from build123d import *

# Parameters (mm, degrees)
SKETCH1_W                      = 132.1
SKETCH1_H                      = 36
BOSS_EXTRUDE1_DEPTH            = 44
CUT_EXTRUDE1_REACH             = 89.147
CUT_EXTRUDE2_REACH             = 89.147
SKETCH3_4_W                    = 23.05
SKETCH3_4_H                    = 12
SKETCH3_4_W_2                  = 52.5
SKETCH3_4_H_2                  = 26
CUT_EXTRUDE3_DEPTH             = 12.5
CUT_EXTRUDE6_DEPTH             = 7.5
CUT_EXTRUDE7_REACH             = 101.054
CUT_EXTRUDE8_REACH             = 137.7
SKETCH11_R                     = 2.55
CUT_EXTRUDE8_DIRECTION_2_REACH = 137.7
SKETCH11_6_R                   = 4.6
SKETCH11_6_R_2                 = 2.55
CUT_EXTRUDE10_DEPTH            = 2.2
CUT_EXTRUDE11_START            = 123.73
SKETCH11_7_R                   = 4.6
SKETCH11_7_R_2                 = 2.55
CUT_EXTRUDE11_DEPTH            = 2.2


with BuildPart() as part:
    # Sketch1 → Boss-Extrude1 (new body)
    with BuildSketch(Plane(origin=(0, 0, 0), x_dir=(1, 0, 0), z_dir=(0, 1, 0))):
        Rectangle(SKETCH1_W, SKETCH1_H)
        Polygon((-57.05, 14.5), (-57.05, -5.5), (20.85, -5.5), (20.85, -3.2), (26.85, 0.267693758), (32.85, -3.2), (33.05, -3.2), (33.05, 9.51), (32.85, 9.51), (26.85, 6.042306242), (20.85, 9.51), (20.85, 13), (-37.95, 13), (-37.95, 14.5), align=None, mode=Mode.SUBTRACT)
    extrude(amount=-BOSS_EXTRUDE1_DEPTH)

    # Cut-Extrude1: up to this face of the body (flat: up to its plane)
    cut_extrude1_end = Plane(part.part.faces().sort_by_distance((0, -22, 18))[0])
    # Sketch3 → Cut-Extrude1 (cut, up to the picked face)
    with BuildSketch(Plane(origin=(0, 0, -18), x_dir=(-1, 0, 0), z_dir=(0, 0, -1)), mode=Mode.PRIVATE) as cut_extrude1_sk1:
        Polygon((-60.48, -18), (-60.48, -44), (-20.85, -44), (-20.85, -29), (-38.35, -29), (-38.35, -22), (-46.35, -14), (-56.48, -14), align=None)
    cut_extrude1_tool1 = split(extrude(cut_extrude1_sk1.sketch, amount=-CUT_EXTRUDE1_REACH, mode=Mode.PRIVATE), bisect_by=cut_extrude1_end, keep=Keep.BOTH, mode=Mode.PRIVATE)
    add(cut_extrude1_tool1.solids().sort_by(Axis((43.76231, -31.789655, -18), (0, 0, 1)))[0], mode=Mode.SUBTRACT)

    # Cut-Extrude2: up to this face of the body (flat: up to its plane)
    cut_extrude2_end = Plane(part.part.faces().sort_by_distance((-18.1, -22, 5.5))[0])
    # Sketch3<4> → Cut-Extrude2 (cut, up to the picked face)
    with BuildSketch(Plane(origin=(0, 0, -18), x_dir=(-1, 0, 0), z_dir=(0, 0, -1)), mode=Mode.PRIVATE) as cut_extrude2_sk1:
        with Locations((20.075, -10.36)):
            Rectangle(SKETCH3_4_W, SKETCH3_4_H)
    cut_extrude2_tool1 = split(extrude(cut_extrude2_sk1.sketch, amount=-CUT_EXTRUDE2_REACH, mode=Mode.PRIVATE), bisect_by=cut_extrude2_end, keep=Keep.BOTH, mode=Mode.PRIVATE)
    # Sketch3<4> → Cut-Extrude2 (cut, up to the picked face)
    with BuildSketch(Plane(origin=(0, 0, -18), x_dir=(-1, 0, 0), z_dir=(0, 0, -1)), mode=Mode.PRIVATE) as cut_extrude2_sk2:
        with Locations((34.8, -31)):
            Rectangle(SKETCH3_4_W_2, SKETCH3_4_H_2)
    cut_extrude2_tool2 = split(extrude(cut_extrude2_sk2.sketch, amount=-CUT_EXTRUDE2_REACH, mode=Mode.PRIVATE), bisect_by=cut_extrude2_end, keep=Keep.BOTH, mode=Mode.PRIVATE)
    add(cut_extrude2_tool1.solids().sort_by(Axis((-20.075, -10.36, -18), (0, 0, 1)))[0], mode=Mode.SUBTRACT)
    add(cut_extrude2_tool2.solids().sort_by(Axis((-34.8, -31, -18), (0, 0, 1)))[0], mode=Mode.SUBTRACT)

    # Sketch4 → Cut-Extrude3 (cut)
    with BuildSketch(Plane.XY.offset(18)):
        Polygon((-61.05, -44), (-61.05, -18), (-57.05, -18), (-57.05, -14), (-35.05, -14), (-27.05, -22), (-27.05, -29), (-14.05, -29), (-5.05, -21.5), (20.85, -21.5), (20.85, -29), (20.85, -44), align=None)
    extrude(amount=-CUT_EXTRUDE3_DEPTH, mode=Mode.SUBTRACT)

    # Sketch7 → Cut-Extrude6 (cut)
    with BuildSketch(Plane.XZ.offset(29)):
        Polygon((20.85, 3.2), (23.35, 5.7), (23.35, 8), (29.35, 8), (28.95, 18), (20.85, 18), align=None)
    extrude(amount=-CUT_EXTRUDE6_DEPTH, mode=Mode.SUBTRACT)

    # Cut-Extrude7: up to this face of the body (flat: up to its plane)
    cut_extrude7_end = Plane(part.part.faces().sort_by_distance((33.05, -14.5, -3.155))[0])
    # Sketch10 → Cut-Extrude7 (cut, up to the picked face)
    with BuildSketch(Plane.ZY.offset(-20.85), mode=Mode.PRIVATE) as cut_extrude7_sk1:
        Polygon((-8.552306242, 0), (-6.042306242, 0), (-6.042306242, -2.51), align=None)
    cut_extrude7_tool1 = split(extrude(cut_extrude7_sk1.sketch, amount=-CUT_EXTRUDE7_REACH, mode=Mode.PRIVATE), bisect_by=cut_extrude7_end, keep=Keep.BOTH, mode=Mode.PRIVATE)
    # Sketch10 → Cut-Extrude7 (cut, up to the picked face)
    with BuildSketch(Plane.ZY.offset(-20.85), mode=Mode.PRIVATE) as cut_extrude7_sk2:
        Polygon((-0.267693758, 0), (-0.267693758, -2.51), (2.242306242, 0), align=None)
    cut_extrude7_tool2 = split(extrude(cut_extrude7_sk2.sketch, amount=-CUT_EXTRUDE7_REACH, mode=Mode.PRIVATE), bisect_by=cut_extrude7_end, keep=Keep.BOTH, mode=Mode.PRIVATE)
    # Sketch10 → Cut-Extrude7 (cut, up to the picked face)
    with BuildSketch(Plane.ZY.offset(-20.85), mode=Mode.PRIVATE) as cut_extrude7_sk3:
        Polygon((-9.51, -29), (-6.042306242, -25.532306242), (-6.042306242, -29), align=None)
    cut_extrude7_tool3 = split(extrude(cut_extrude7_sk3.sketch, amount=-CUT_EXTRUDE7_REACH, mode=Mode.PRIVATE), bisect_by=cut_extrude7_end, keep=Keep.BOTH, mode=Mode.PRIVATE)
    # Sketch10 → Cut-Extrude7 (cut, up to the picked face)
    with BuildSketch(Plane.ZY.offset(-20.85), mode=Mode.PRIVATE) as cut_extrude7_sk4:
        Polygon((-0.267693758, -25.532306242), (-0.267693758, -29), (3.2, -29), align=None)
    cut_extrude7_tool4 = split(extrude(cut_extrude7_sk4.sketch, amount=-CUT_EXTRUDE7_REACH, mode=Mode.PRIVATE), bisect_by=cut_extrude7_end, keep=Keep.BOTH, mode=Mode.PRIVATE)
    add(cut_extrude7_tool1.solids().sort_by(Axis((20.85, -0.836667, -6.878973), (1, 0, 0)))[0], mode=Mode.SUBTRACT)
    add(cut_extrude7_tool2.solids().sort_by(Axis((20.85, -0.836667, 0.568973), (1, 0, 0)))[0], mode=Mode.SUBTRACT)
    add(cut_extrude7_tool3.solids().sort_by(Axis((20.85, -27.844102, -7.198204), (1, 0, 0)))[0], mode=Mode.SUBTRACT)
    add(cut_extrude7_tool4.solids().sort_by(Axis((20.85, -27.844102, 0.888204), (1, 0, 0)))[0], mode=Mode.SUBTRACT)

    # Cut-Extrude8: up to this face of the body (flat: up to its plane)
    cut_extrude8_end = Plane(part.part.faces().sort_by_distance((-66.05, -22, 0))[0])
    # Sketch11 → Cut-Extrude8 (cut, up to the picked face)
    with BuildSketch(Plane(origin=(-61.05, 0, 0), x_dir=(0, 0, -1), z_dir=(1, 0, 0)), mode=Mode.PRIVATE) as cut_extrude8_sk1:
        with Locations((-8, -34)):
            Circle(SKETCH11_R)
    cut_extrude8_tool1 = split(extrude(cut_extrude8_sk1.sketch, amount=-CUT_EXTRUDE8_REACH, mode=Mode.PRIVATE), bisect_by=cut_extrude8_end, keep=Keep.BOTH, mode=Mode.PRIVATE)
    # Sketch11 → Cut-Extrude8 (cut, up to the picked face)
    with BuildSketch(Plane(origin=(-61.05, 0, 0), x_dir=(0, 0, -1), z_dir=(1, 0, 0)), mode=Mode.PRIVATE) as cut_extrude8_sk2:
        with Locations((8, -34)):
            Circle(SKETCH11_R)
    cut_extrude8_tool2 = split(extrude(cut_extrude8_sk2.sketch, amount=-CUT_EXTRUDE8_REACH, mode=Mode.PRIVATE), bisect_by=cut_extrude8_end, keep=Keep.BOTH, mode=Mode.PRIVATE)
    add(cut_extrude8_tool1.solids().sort_by(Axis((-61.05, -34, 8), (-1, 0, 0)))[0], mode=Mode.SUBTRACT)
    add(cut_extrude8_tool2.solids().sort_by(Axis((-61.05, -34, -8), (-1, 0, 0)))[0], mode=Mode.SUBTRACT)

    # Cut-Extrude8 direction 2: up to this face of the body (flat: up to its plane)
    cut_extrude8_direction_2_end = Plane(part.part.faces().sort_by_distance((66.05, -22, 0))[0])
    # Sketch11 → Cut-Extrude8 direction 2 (cut, up to the picked face)
    with BuildSketch(Plane(origin=(-61.05, 0, 0), x_dir=(0, 0, -1), z_dir=(1, 0, 0)), mode=Mode.PRIVATE) as cut_extrude8_direction_2_sk1:
        with Locations((-8, -34)):
            Circle(SKETCH11_R)
    cut_extrude8_direction_2_tool1 = split(extrude(cut_extrude8_direction_2_sk1.sketch, amount=CUT_EXTRUDE8_DIRECTION_2_REACH, mode=Mode.PRIVATE), bisect_by=cut_extrude8_direction_2_end, keep=Keep.BOTH, mode=Mode.PRIVATE)
    # Sketch11 → Cut-Extrude8 direction 2 (cut, up to the picked face)
    with BuildSketch(Plane(origin=(-61.05, 0, 0), x_dir=(0, 0, -1), z_dir=(1, 0, 0)), mode=Mode.PRIVATE) as cut_extrude8_direction_2_sk2:
        with Locations((8, -34)):
            Circle(SKETCH11_R)
    cut_extrude8_direction_2_tool2 = split(extrude(cut_extrude8_direction_2_sk2.sketch, amount=CUT_EXTRUDE8_DIRECTION_2_REACH, mode=Mode.PRIVATE), bisect_by=cut_extrude8_direction_2_end, keep=Keep.BOTH, mode=Mode.PRIVATE)
    add(cut_extrude8_direction_2_tool1.solids().sort_by(Axis((-61.05, -34, 8), (1, 0, 0)))[0], mode=Mode.SUBTRACT)
    add(cut_extrude8_direction_2_tool2.solids().sort_by(Axis((-61.05, -34, -8), (1, 0, 0)))[0], mode=Mode.SUBTRACT)

    # Sketch11<6> → Cut-Extrude10 (cut)
    # profile 1 of 2: a face of its own
    with BuildSketch(Plane(origin=(-61.05, 0, 0), x_dir=(0, 0, -1), z_dir=(1, 0, 0))):
        with Locations((-8, -34)):
            Circle(SKETCH11_6_R)
        with Locations((-8, -34)):
            Circle(SKETCH11_6_R_2, mode=Mode.SUBTRACT)
    # profile 2 of 2: a face of its own
    with BuildSketch(Plane(origin=(-61.05, 0, 0), x_dir=(0, 0, -1), z_dir=(1, 0, 0))):
        with Locations(Location((8, -34, 0), (0, 0, 180))):
            Circle(SKETCH11_6_R)
        with Locations(Location((8, -34, 0), (0, 0, 180))):
            Circle(SKETCH11_6_R_2, mode=Mode.SUBTRACT)
    extrude(amount=-CUT_EXTRUDE10_DEPTH, mode=Mode.SUBTRACT)

    # Sketch11<7> → Cut-Extrude11 (cut)
    # profile 1 of 2: a face of its own
    with BuildSketch(Plane(origin=(-61.05, 0, 0), x_dir=(0, 0, -1), z_dir=(1, 0, 0)).offset(CUT_EXTRUDE11_START)):
        with Locations((-8, -34)):
            Circle(SKETCH11_7_R)
        with Locations((-8, -34)):
            Circle(SKETCH11_7_R_2, mode=Mode.SUBTRACT)
    # profile 2 of 2: a face of its own
    with BuildSketch(Plane(origin=(-61.05, 0, 0), x_dir=(0, 0, -1), z_dir=(1, 0, 0)).offset(CUT_EXTRUDE11_START)):
        with Locations(Location((8, -34, 0), (0, 0, 180))):
            Circle(SKETCH11_7_R)
        with Locations((8, -34)):
            Circle(SKETCH11_7_R_2, mode=Mode.SUBTRACT)
    extrude(amount=-CUT_EXTRUDE11_DEPTH, mode=Mode.SUBTRACT)


solid = part.part
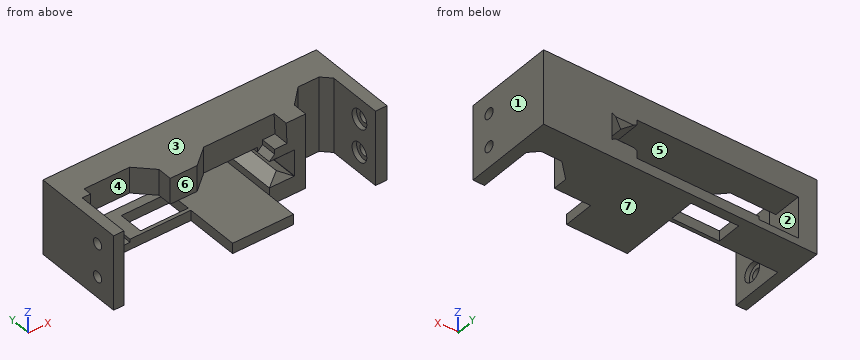
The model under review builds one solid part; all positions refer to its coordinate system, in mm. Face numbers are marked on the shaded views. A direction names the side the tool comes from. Round coordinates to 2 decimals unless told otherwise and drop trailing zeros. Order: outer loops, then holes, each group sorted by start corner. A loop starts at its lowest first (then second) coordinate and runs counter-clockwise, first axis right, second up. Notation, with made-up numbers: (-29.75, 25.5) -> (-11.75, 25.5) arc R14 ccw to (-11.75, 52.5) -> close; hole circle Ø2 at (14, -26). An arc over 180 degrees is marked (long way). Return JSON: item names as keys, results as strings.
1. Take a section at A-A (x = 17.5). Write out the cut boundary in (y, z), then the cut area to 3 significant figures.
Answer block:
{"outline": "(-44, -18) -> (0, -18) -> (0, -13) -> (-44, -13) -> close; (-21.5, 5.5) -> (0, 5.5) -> (0, 18) -> (-21.5, 18) -> close", "area": "489 mm²"}
2. For L1, parallel to X at y = -26.5, z = -16; L2, parallel to Y at x = -61.45, z = 8; L3, parallel to X at y = -24, z = -2, list the stretches that pass through material, from the lowest coordinate up. Write a range as [from, to].
Answer block:
{"L1": "x = [-66.05, -61.05], [-8.55, 38.35], [60.48, 66.05]", "L2": "y = [-44, -38.6], [-29.4, 0]", "L3": "x = [-66.05, -61.05], [33.05, 38.35], [60.48, 66.05]"}
3. The part is to be moulded in two halves that separate along Z. For the marked faces 1, 2 and 3, say which applies: +Z half, -Z half, draft (parallel to the pull), parting line (faces both ways), or undercut.
Answer block:
{"face 1": "draft", "face 2": "undercut", "face 3": "+Z half"}
4. Take a section at C-C (z = 1). Write out the cut boundary in (x, y), then the cut area to 3 significant figures.
Answer block:
{"outline": "(-66.05, -44) -> (-61.05, -44) -> (-61.05, -18) -> (-57.05, -18) -> (-57.05, 0) -> (-66.05, 0) -> close; (24.66, -26.8) -> (29.04, -26.8) -> (29.04, -1.24) -> (24.66, -1.24) -> close; (33.05, -29) -> (38.35, -29) -> (38.35, -22) -> (46.35, -14) -> (56.48, -14) -> (60.48, -18) -> (60.48, -44) -> (66.05, -44) -> (66.05, 0) -> (33.05, 0) -> close", "area": "1,150 mm²"}
5. Take a section at B-B (y = -6). Write out the cut boundary in (x, z).
Answer block:
{"outline": "(-66.05, -18) -> (-31.6, -18) -> (-31.6, -13) -> (-37.95, -13) -> (-37.95, -14.5) -> (-57.05, -14.5) -> (-57.05, 5.5) -> (20.85, 5.5) -> (20.85, 3.2) -> (26.85, -0.27) -> (32.85, 3.2) -> (33.05, 3.2) -> (33.05, -9.51) -> (32.85, -9.51) -> (26.85, -6.04) -> (20.85, -9.51) -> (20.85, -13) -> (-8.55, -13) -> (-8.55, -18) -> (66.05, -18) -> (66.05, 18) -> (-66.05, 18) -> close"}
6. Take a section at D-D (y = -34). State how many separate pieces and enclosed holes the cut face has, then the cut area to 3 significant figures.
Answer block:
{"separate pieces": "7", "enclosed holes": "0", "area": "384 mm²"}
7. For the marked faces 4, 5, 6 and 7, list the 3-axis set-ups (+Z, -Z, +X, -X, +Y, -Y) from which the entire face can be reached by the end or side of a thin tool; tool diameter is ignored.
Answer block:
{"face 4": "+Z, -Y", "face 5": "+Y, -Y", "face 6": "+Z, -Z, -Y", "face 7": "-Z, +X, -X, +Y, -Y"}
8. Insertion check: P1, Ø6, axis at x = -40, y = -17.5, coming from the +Z side; P2, Ø14.5, axis at y = -34, z = 8, coming from the -X side; P3, Ø2.5, axis at x = -25, z = -14.5, coming from the -Y side; P4, Ø12, axis at x = 33.5, z = 13.5, coming from the -Y side. Each pin has a flat end and moves straight along its axis. Give the tip position at first contact, or say it passes through.
Answer block:
{"P1": "stops at z = -13", "P2": "stops at x = -66.05", "P3": "stops at y = -18", "P4": "stops at y = -29"}
